from build123d import *

# Parameters (mm, degrees)
F1_DEPTH = 5
F3_D     = 4.2
F3_DEPTH = 12.4
F3_TIP   = 1.2618073
F5_D     = 4.2
F5_DEPTH = 12.4
F5_TIP   = 1.2618073


# Not quite as in the source:
# - a feature names something its author has since deleted; it is built from what else it names


with BuildPart() as f1:
    # F0 (on Front) → F1 (new body, symmetric)
    with BuildSketch(Plane.XZ):
        Polygon((0, 90), (0, 0), (58, 0), (58, 30), (20, 90), align=None)
    extrude(amount=F1_DEPTH, both=True)

    # F3
    with Locations(Plane(origin=(0, 0, 0), x_dir=(1, 0, 0), z_dir=(0, 0, -1))):
        with Locations((26, 0), (48, 0)):
            Hole(F3_D / 2, depth=F3_DEPTH)
            with Locations((0, 0, -(F3_DEPTH + F3_TIP / 2))):  # 118° drill point
                Cone(0, F3_D / 2, F3_TIP, mode=Mode.SUBTRACT)

    # F5
    with Locations(Plane(origin=(0, 0, 0), x_dir=(0, -1, 0), z_dir=(-1, 0, 0))):
        with Locations((0, 20), (0, 82), (0, 51)):
            Hole(F5_D / 2, depth=F5_DEPTH)
            with Locations((0, 0, -(F5_DEPTH + F5_TIP / 2))):  # 118° drill point
                Cone(0, F5_D / 2, F5_TIP, mode=Mode.SUBTRACT)


solid = f1.part
Source: CAD feature listing. Evaluate the final solid. Frame: model axes, mm. A direction names the side the tool comes from. Give positions to 0.01 mm unless a question says otherwise; leave off trailing zeros. Write each loop counter-clockwise with the first axis right and the second up, starting at its lowest first coordinate (ties: lowest second). Pieces come first, ordered by that corner, then holes. Notation, with made-up numbers: (39.5, 46.25) -> (46.5, 46.25) arc R15 ccw to (46.5, 53.25) -> close; hole circle Ø1 at (71.25, 69). An arc over 180 degrees is marked (long way). Return JSON: item names as keys, results as strings. Group by question number.
1. Section D-D, the plane x = 33. Output: boundary loops of the cut face in (y, z), then the cut area to 3 significant figures.
2. Section C-C, the plane y = 3.75. Output: boundary loops of the cut face in (x, z), then the cut area to 3 significant figures.
3. Material intervals for line 1 (Z direction, x = 3.5, y = 0); line 2 (Y direction, x = 26, z = 4.5); line 3 (Z direction, x = 5.5, y = 1.5), sorted ascending. Write a range as from..to.
4. Section A-A, the plane x = 7.5. Output: boundary loops of the cut face in (y, z).
5. Access query for faces 1 (the face through (29, 0, 0)), 2 (the face through (6.287, -1.666, 80.722)), 3 (the face through (46.06, 0.8, 6.29)). Directions: +Z, -Z, +X, -X, +Y, -Y. A direction counts if a zero-diameter tool reaches every point of the face in a straight line with its end or side. Return the directions, or none.
6. Pin query (flat end, axial travel): pin 1 Ø2.5 at (x, y) = (48, 0) entering from +Z; pin 2 Ø1 at (x, y) = (43, -1) entering from -Z; pin 3 Ø4 at (x, y) = (23.5, 3) entering from +Z; pin 4 Ø4 at (y, z) = (0, 82) entering from -X. Return the tip coordinate at first contact, or that it passes through.
7. Section B-B, the plane z = 7.5. Output: boundary loops of the cut face in (x, y), then the cut area to 3 significant figures.
8. Mould query, pull axis Z, two halves, no side actions, for faces 4 (the face through (22, 5, 36)), 5 (the face through (13.44, -0.2, 51.31)), 6 (the face through (10, 0, 90)), 7 (the face through (13.44, 0.08, 19.64)). Classes: +Z half, -Z half, draft (parallel to the pull), parting line (faces both ways), or undercut.
Determined:
{
 "1": {"outline": "(-5, 0) -> (5, 0) -> (5, 69.47) -> (-5, 69.47) -> close", "area": "695 mm2"},
 "2": {"outline": "(0, 0) -> (58, 0) -> (58, 30) -> (20, 90) -> (0, 90) -> close", "area": "4,080 mm2"},
 "3": {"line 1": "z = 0..17.9, 22.1..48.9, 53.1..79.9, 84.1..90", "line 2": "y = -5..-2.1, 2.1..5", "line 3": "z = 0..18.53, 21.47..49.53, 52.47..80.53, 83.47..90"},
 "4": {"outline": "(-5, 0) -> (5, 0) -> (5, 90) -> (-5, 90) -> close; hole circle Ø4.2 at (0, 20); hole circle Ø4.2 at (0, 51); hole circle Ø4.2 at (0, 82)"},
 "5": {"face 1": "-Z, +X, -X, +Y, -Y", "face 2": "-X", "face 3": "-Z"},
 "6": {"pin 1": "stops at z = 47.76", "pin 2": "stops at z = 0", "pin 3": "stops at z = 87.63", "pin 4": "stops at x = 12.46"},
 "7": {"outline": "(0, -5) -> (58, -5) -> (58, 5) -> (0, 5) -> close; hole circle Ø4.2 at (26, 0); hole circle Ø4.2 at (48, 0)", "area": "552 mm2"},
 "8": {"face 4": "draft", "face 5": "undercut", "face 6": "+Z half", "face 7": "undercut"}
}
